Could you check a few things on this model? Use its own coordinates, in mm. A direction names the side the tool comes from. Give positions to 0.01 mm unless a question says otherwise; leave off trailing zeros. Order: outer loops, then holes, each group sorted by start corner. A loop starts at its lowest first (then second) coordinate and runs counter-clockwise, first axis right, second up. Notation, with made-up numbers: M 17.5,22 L 47.5,22 A23 cw 47.5,52 Z; hole C 0.25,42 d5. An arc over 180 degrees is marked long. Answer in a Markdown table with one row per item. Add a question column.
```python
from build123d import *

# Parameters (mm, degrees)
BOSS_EXTRUDE1_DEPTH = 15
SKETCH1_3_R         = 5
SKETCH1_3_R_2       = 10
CUT_EXTRUDE1_DEPTH  = 15
BOSS_EXTRUDE2_DEPTH = 25
CUT_EXTRUDE3_DEPTH  = 254.673017879


with BuildPart() as part:
    # Sketch1 → Boss-Extrude1 (new body)
    with BuildSketch(Plane.XY):
        Polygon((-35, 150), (35, 150), (35, 110), (30, 95), (30, -95), (35, -110), (35, -150), (-35, -150), (-35, -110), (-30, -95), (-30, 95), (-35, 110), align=None)
    extrude(amount=-BOSS_EXTRUDE1_DEPTH)

    # Sketch1_3 → Cut-Extrude1 (cut)
    with BuildSketch(Plane.XY):
        with Locations((-20, 130)):
            Circle(SKETCH1_3_R)
        with Locations(Location((20, 130, 0), (0, 0, 180))):
            Circle(SKETCH1_3_R)
        with Locations((0, -80)):
            Circle(SKETCH1_3_R_2)
        with Locations((20, -130)):
            Circle(SKETCH1_3_R)
        with Locations(Location((-20, -130, 0), (0, 0, 180))):
            Circle(SKETCH1_3_R)
    extrude(amount=-CUT_EXTRUDE1_DEPTH, mode=Mode.SUBTRACT)

    # Sketch1_4 → Boss-Extrude2 (add)
    with BuildSketch(Plane.XY):
        with BuildLine():
            Line((-17.5, 100), (17.5, 100))
            ThreePointArc((17.5, 100), (18.207106781, 99.707106781), (18.5, 99))
            Line((18.5, 99), (18.5, 94))
            ThreePointArc((18.5, 94), (18.207106781, 93.292893219), (17.5, 93))
            Line((17.5, 93), (-17.5, 93))
            ThreePointArc((-17.5, 93), (-18.207106781, 93.292893219), (-18.5, 94))
            Line((-18.5, 94), (-18.5, 99))
            ThreePointArc((-18.5, 99), (-18.207106781, 99.707106781), (-17.5, 100))
        make_face()
        with BuildLine():
            Line((-17.5, 68), (17.5, 68))
            ThreePointArc((17.5, 68), (18.207106781, 67.707106781), (18.5, 67))
            Line((18.5, 67), (18.5, 62))
            ThreePointArc((18.5, 62), (18.207106781, 61.292893219), (17.5, 61))
            Line((17.5, 61), (-17.5, 61))
            ThreePointArc((-17.5, 61), (-18.207106781, 61.292893219), (-18.5, 62))
            Line((-18.5, 62), (-18.5, 67))
            ThreePointArc((-18.5, 67), (-18.207106781, 67.707106781), (-17.5, 68))
        make_face()
    extrude(amount=BOSS_EXTRUDE2_DEPTH)

    # Sketch2 → Cut-Extrude3 (cut, through all)
    with BuildSketch(Plane(origin=(0, 100, 0), x_dir=(1, 0, 0), z_dir=(0, 1, 0))):
        with BuildLine():
            Line((-6.5, -8.758342613), (-6.5, -16.241657387))
            ThreePointArc((-6.5, -16.241657387), (0, -20), (6.5, -16.241657387))
            Line((6.5, -16.241657387), (6.5, -8.758342613))
            ThreePointArc((6.5, -8.758342613), (0, -5), (-6.5, -8.758342613))
        make_face()
    extrude(amount=-CUT_EXTRUDE3_DEPTH, mode=Mode.SUBTRACT)


solid = part.part
```
1. Will these pins go through, and if not, where does the flat tip stop? P1, Ø10, axis at x = -21.5, z = 7, coming from the -Y side; P2, Ø7.5, axis at y = 29.5, z = -5, coming from the -X side; P3, Ø2, axis at y = 98, z = 14, coming from the -X side.
2. For faces 4 (the cylindrical face through (0, 65, 5)), 5 (the flat face through (30, 1, -7)), 6 (the flat face through (-18.5, 96, 12)), which set-ups out of +Z, -Z, +X, -X, +Y, -Y let a thin tool reach every point of the face, with its end or its side?
3. Thinking about a two-plate mould opening in Y: for faces 1 (the flat face through (6.5, 65, 13)), 2 (the flat face through (0, -150, -7)), 3 (the flat face through (32.535, 102.605, -7.395)), which applies, pulls with the +Y half, pulls with the -Y half, needs draft (parallel to the pull), parting line crosses it, or undercut?
4. If I drill on line 1 along Y through (x, z) = (20, -4); line 2 along Y through (x, z) = (-12, 8); line 3 along Y through (x, z) = (21.5, -5.5), over which ranges is the centre line in solid material (lowest first)? Write a range as [from, to].
5. Suppose I cut it at D-D on x = 21. List the corners of the cut face in (y, z) for me.
6. Suppose I cut it at B-B on z = -6. List the corners of the cut face in (x, y) for me, plus the area to 3 significant figures.
7. Suppose I cut it at C-C on y = 130. List the corners of the cut face in (x, z) for me, plus the area to 3 significant figures.
8. Suppose I cut it at A-A on x = 0. List the corners of the cut face in (y, z) for me, plus the area to 3 significant figures.
Findings below:
| question | item | result |
|---|---|---|
| 1 | P1 | y = 61 |
| 1 | P2 | x = -30 |
| 1 | P3 | x = -18.5 |
| 2 | face 4 | +Y, -Y |
| 2 | face 5 | +Z, -Z, +X |
| 2 | face 6 | +Z, -X, +Y, -Y |
| 3 | face 1 | needs draft |
| 3 | face 2 | pulls with the -Y half |
| 3 | face 3 | undercut |
| 4 | line 1 | [-150, -135], [-125, 125], [135, 150] |
| 4 | line 2 | [61, 68], [93, 100] |
| 4 | line 3 | [-150, -134.77], [-125.23, 125.23], [134.77, 150] |
| 5 | outline | M -150,-15 L -134.9,-15 L -134.9,0 L -150,0 Z; M -125.1,-15 L 125.1,-15 L 125.1,0 L -125.1,0 Z; M 134.9,-15 L 150,-15 L 150,0 L 134.9,0 Z |
| 6 | outline | M -35,-150 L 35,-150 L 35,-110 L 30,-95 L 30,95 L 35,110 L 35,150 L -35,150 L -35,110 L -30,95 L -30,-95 L -35,-110 Z; hole C -20,-130 d10; hole C -20,130 d10; hole C 0,-80 d20; hole C 20,-130 d10; hole C 20,130 d10 |
| 6 | area | 18,300 mm2 |
| 7 | outline | M -35,-15 L -25,-15 L -25,0 L -35,0 Z; M -15,-15 L 15,-15 L 15,0 L -15,0 Z; M 25,-15 L 35,-15 L 35,0 L 25,0 Z |
| 7 | area | 750 mm2 |
| 8 | outline | M -150,-15 L -90,-15 L -90,0 L -150,0 Z; M -70,-15 L 150,-15 L 150,0 L 100,0 L 100,5 L 93,5 L 93,0 L 68,0 L 68,5 L 61,5 L 61,0 L -70,0 Z; M 61,20 L 68,20 L 68,25 L 61,25 Z; M 93,20 L 100,20 L 100,25 L 93,25 Z |
| 8 | area | 4,340 mm2 |
